```python
from build123d import *

# Parameters (mm, degrees)
SKETCH1_W = 15
SKETCH1_H = 25
FILLET1_R = 5
FILLET2_R = 0.5


with BuildPart() as part:
    # Sketch1 → Revolve1 (revolve)
    with BuildSketch(Plane.YZ, mode=Mode.PRIVATE) as revolve1_sk:
        with Locations((7.5, 0)):
            Rectangle(SKETCH1_W, SKETCH1_H)
    revolve(revolve1_sk.sketch.rotate(Axis((0, 0, 22.327044025), (0, 0, -1)), 180), axis=Axis((0, 0, 22.327044025), (0, 0, -1)))

    # Fillet1
    fillet1_edges = [part.edges().sort_by_distance(p)[0] for p in [
        (0, 15, 12.5),
    ]]
    fillet(fillet1_edges, radius=FILLET1_R)

    # Fillet2
    fillet2_edges = [part.edges().sort_by_distance(p)[0] for p in [
        (0, 15, -12.5),
    ]]
    fillet(fillet2_edges, radius=FILLET2_R)


solid = part.part
```
CAD build for the part. Positions are in the model's coordinates, mm. Round coordinates to 2 decimals unless told otherwise and drop trailing zeros. Loops run counter-clockwise (first coordinate to the right, second up) from the corner with the lowest first, then second, coordinate; pieces in that order, holes last. Notation, with made-up numbers: M 38.25,-31 L 60.25,-31 A26 cw 60.25,-13 Z; hole C 32.25,-27.5 d2. An arc over 180 degrees is marked long. Use a Markdown table: item, result. Add a question column.
(1) Cut at A-A (z = 0). Give the cut face in (x, y), and give its area (3 significant figures).
(2) Flat gauge pins, fed straight in: pin 1 (12 mm diameter, centred on y = -11, z = -6, fed in from +X); pin 2 (10 mm diameter, centred on x = 5.5, z = 7, fed in from -Y); pin 3 (8 mm diameter, centred on x = -4.5, z = -5, fed in from +Y). Where does each tip first touch, or does it go through?
(3) Drill centre lines: line 1 (Z direction, x = 1.25, y = -10); line 2 (X direction, y = -0.5, z = 5.25); line 3 (X direction, y = 2.5, z = -7.5). Where is each one in solid material? Low to high.
(4) Cut at B-B (z = 9.25). Give the cut face in (x, y), and give its area (3 significant figures).
Geometry says:
| question | item | result |
|---|---|---|
| 1 | outline | C 0,0 d30 |
| 1 | area | 707 mm² |
| 2 | pin 1 | stops at x = 14.14 |
| 2 | pin 2 | stops at y = -14.99 |
| 2 | pin 3 | stops at y = 14.99 |
| 3 | line 1 | z = -12.5 to 12.5 |
| 3 | line 2 | x = -14.99 to 14.99 |
| 3 | line 3 | x = -14.79 to 14.79 |
| 4 | outline | C 0,0 d29.37 |
| 4 | area | 677 mm² |
